Autodesk Inventor part; units mm, degrees
ref_plane "YZ Plane" through (0, 0, 0) normal (1, 0, 0) x (0, 1, 0)
ref_plane "XZ Plane" through (0, 0, 0) normal (0, 1, 0) x (-1, 0, 0)
ref_plane "XY Plane" through (0, 0, 0) normal (0, 0, 1) x (1, 0, 0)
sketch "Sketch1" plane through (0, 0, 0) normal (0, 1, 0) x (-1, 0, 0)
  line L0 (0, 0) -> (25.4, 0)
  line L1 (25.4, 0) -> (25.4, -25.4)
  line L2 (25.4, -25.4) -> (0, -25.4)
  line L3 (0, -25.4) -> (0, 0)
  line L4 (23.8125, -23.8125) -> (23.8125, -1.5875)
  line L5 (23.8125, -1.5875) -> (1.5875, -1.5875)
  line L6 (1.5875, -1.5875) -> (1.5875, -23.8125)
  line L7 (1.5875, -23.8125) -> (23.8125, -23.8125)
  dimension "d0" = 25.4
  dimension "d1" = 25.4
  dimension "d2" = 1.5875
extrude "Extrusion1" add sketch "Sketch1" along normal blind 405.9428
sketch "Sketch4" plane through (-25.4, 0, 0) normal (0, 0, 1) x (1, 0, 0)
  circle A0 centre (12.7, 177.8) radius 6.35
  line L0 (0, 0) -> (0, 405.9428)
  line L1 (25.4, 0) -> (0, 0)
  dimension "d13" = 12.7
  dimension "d14" = 12.7
  dimension "d15" = 177.8
extrude "Extrusion4" cut sketch "Sketch4" against normal blind 25.4
sketch "Sketch5" plane through (0, 0, 0) normal (0, -1, 0) x (1, 0, 0)
  line L0 (-25.4, -25.4) -> (0, -25.4)
  line L1 (0, 0) -> (-25.4, 0)
  line L2 (-25.4, -25.4) -> (0, -25.4)
  line L3 (0, -25.4) -> (0, 0)
  line L4 (0, 0) -> (-25.4, 0)
  line L5 (-25.4, 0) -> (-25.4, -25.4)
  line L6 (-23.8125, -1.5875) -> (-1.5875, -1.5875)
  line L7 (-23.8125, -23.8125) -> (-23.8125, -1.5875)
  line L8 (-1.5875, -1.5875) -> (-23.8125, -1.5875)
  line L9 (-23.8125, -1.5875) -> (-23.8125, -23.8125)
  line L10 (-23.8125, -23.8125) -> (-1.5875, -23.8125)
  line L11 (-1.5875, -23.8125) -> (-1.5875, -1.5875)
extrude "Extrusion5" add sketch "Sketch5" along normal blind 38.1
sketch "Sketch6" plane through (-25.4, 405.9428, 0) normal (0, 0, 1) x (1, 0, 0)
  circle A0 centre (12.7, -431.3428) radius 6.35
  line L0 (25.4, -444.0428) -> (0, -444.0428)
  line L1 (0, 0) -> (0, -444.0428)
  point P0 (25.4, -405.9428)
  dimension "d21" = 12.7
  dimension "d22" = 12.7
  dimension "d23" = 12.7
extrude "Extrusion6" cut sketch "Sketch6" against normal blind 38.1
sketch "Sketch7" plane through (0, 405.9428, -25.4) normal (0, 0, -1) x (-1, 0, 0)
  circle A0 centre (12.7, -12.7) radius 6.35
  line L0 (0, 0) -> (0, -444.0428)
  line L1 (25.4, -444.0428) -> (0, -444.0428)
  line L2 (0, 0) -> (25.4, 0)
  point P0 (0, -405.9428)
  dimension "d26" = 12.7
  dimension "d31" = 12.7
  dimension "d32" = 12.7
extrude "Extrusion7" cut sketch "Sketch7" against normal blind 25.4
properties part number "AP 4"
Design review of the part built by this model. Coordinates are the model's own, in mm. A direction names the side the tool comes from. Round coordinates to 2 decimals unless told otherwise and drop trailing zeros. Write each loop counter-clockwise with the first axis right and the second up, starting at its lowest first coordinate (ties: lowest second). Pieces come first, ordered by that corner, then holes. Notation, with made-up numbers: (85.25, -13) -> (140.25, -13) arc R4 cw to (140.25, -6) -> close; hole circle Ø7 at (62.5, -24). An arc over 180 degrees is marked (long way). One line per question, with ' | ' between items.
(1) Machinability: for faces 1 (the flat face through (-1.588, 187, -13)), 2 (the cylindrical face through (-9.77, -31.034, -0.783)), which of the approach directions +Z, -Z, +X, -X, +Y, -Y give a long, thin tool a straight path to every point of the face, cutting with its end or side? Answer none if there is none.
Result sheet:
face 1: +Y, -Y | face 2: +Z, -Z
(2) Draft analysis for pull direction Z (two halves, no side actions). For faces 3 (the cylindrical face through (-14.08, 171.6, -24.6)), 4 (the flat face through (-13, 187, 0)), 5 (the flat face through (-13, 187, -25.4)), 6 (the flat face through (-13, 187, -23.812)), state which applies: released by +Z, released by -Z, zero draft, split by the parting line, or undercut.
Result sheet:
face 3: zero draft | face 4: released by +Z | face 5: released by -Z | face 6: undercut
(3) Take a section at C-C, the plane z = -18.5. State the section outline as (x, y) points, and give its area (3 significant figures).
Result sheet:
outline: (-25.4, -38.1) -> (-23.81, -38.1) -> (-23.81, 405.94) -> (-25.4, 405.94) -> close; (-1.59, -38.1) -> (0, -38.1) -> (0, 405.94) -> (-1.59, 405.94) -> close | area: 1,410 mm2
(4) Take a section at A-A, the plane x = -12.7. State how many separate pieces and enclosed holes the cut face has, and give its area (3 significant figures).
Result sheet:
separate pieces: 8 | enclosed holes: 0 | area: 1,290 mm2
(5) Wall thickness on line 1 (Y direction, x = -12.7, z = -0.65); line 2 (Z direction, x = -19.5, y = 223.5): over which ranges is each line inside the solid? List them lowest first. Write a range as [from, to].
Result sheet:
line 1: [-38.1, -31.75], [-19.05, 171.45], [184.15, 386.89], [399.59, 405.94] | line 2: [-25.4, -23.81], [-1.59, 0]
(6) Take a section at D-D, the plane y = 79. State the section outline as (x, z) points, and give its area (3 significant figures).
Result sheet:
outline: (-25.4, -25.4) -> (0, -25.4) -> (0, 0) -> (-25.4, 0) -> close; hole (-23.81, -23.81) -> (-1.59, -23.81) -> (-1.59, -1.59) -> (-23.81, -1.59) -> close | area: 151 mm2
(7) Take a section at B-B, the plane y = -25.4. State the section outline as (x, z) points.
Result sheet:
outline: (-25.4, -25.4) -> (-19.05, -25.4) -> (-19.05, -23.81) -> (-23.81, -23.81) -> (-23.81, -1.59) -> (-19.05, -1.59) -> (-19.05, 0) -> (-25.4, 0) -> close; (-6.35, -25.4) -> (0, -25.4) -> (0, 0) -> (-6.35, 0) -> (-6.35, -1.59) -> (-1.59, -1.59) -> (-1.59, -23.81) -> (-6.35, -23.81) -> close
